from build123d import *

# Parameters (mm, degrees)
SKETCH002_W  = 4
SKETCH002_H  = 3
PAD002_DEPTH = 4
SKETCH_W     = 2
SKETCH_H     = 4
PAD_DEPTH    = 6


with BuildPart() as part:
    # Sketch002 → Pad002 (new body)
    with BuildSketch(Plane.XZ.offset(-2)):
        Polygon((3.75, 0), (3.75, 22), (3.75, 22), (2.25, 22), (-3.75, 22), (-3.75, 0), (-3.75, -3.5), (6.25, -3.5), (6.25, -1.5), (-1.75, -1.5), (-1.75, 0), align=None)
        with Locations((0.25, 16.5)):
            Rectangle(SKETCH002_W, SKETCH002_H, mode=Mode.SUBTRACT)
    extrude(amount=PAD002_DEPTH)

    # Sketch (on Pad) → Pad (join)
    with BuildSketch(Plane.XZ.offset(-2)):
        with Locations((-2.75, 13)):
            Rectangle(SKETCH_W, SKETCH_H)
    pad = extrude(amount=PAD_DEPTH)

    # Mirrored: Pad across XZ
    add(pad.mirror(Plane.XZ))


solid = part.part
The model under review builds one solid part; all positions refer to its coordinate system, in mm. A direction names the side the tool comes from. Round coordinates to 2 decimals unless told otherwise and drop trailing zeros. Loops run counter-clockwise (first coordinate to the right, second up) from the corner with the lowest first, then second, coordinate; pieces in that order, holes last. Notation, with made-up numbers: M 54.5,-7 L 108.5,-7 A30 ccw 108.5,19 Z; hole C -2,-15 d2. An arc over 180 degrees is marked long. Answer as a JSON object with one key per item and string values.
Item 1: For line 1 along X through (y, z) = (1.5, 17.25); line 2 along Z through (x, y) = (0.75, 0); line 3 along X through (y, z) = (0.5, 19.25), list the stretches that pass through material, from the lowest coordinate up.
Check sheet entries:
{"line 1": "-3.75 to -1.75, 2.25 to 3.75", "line 2": "-3.5 to -1.5, 0 to 15, 18 to 22", "line 3": "-3.75 to 3.75"}
Item 2: We need section A-A, the plane x = -1. State the section outline as (y, z) points, and give its area (3 significant figures).
Check sheet entries:
{"outline": "M -2,-3.5 L 2,-3.5 L 2,-1.5 L -2,-1.5 Z; M -2,0 L 2,0 L 2,15 L -2,15 Z; M -2,18 L 2,18 L 2,22 L -2,22 Z", "area": "84.0 mm2"}
Item 3: We need section B-B, the plane y = -0.75. State the section outline as (x, z) points, and give its area (3 significant figures).
Check sheet entries:
{"outline": "M -3.75,-3.5 L 6.25,-3.5 L 6.25,-1.5 L -1.75,-1.5 L -1.75,0 L 3.75,0 L 3.75,22 L -3.75,22 Z; hole M -1.75,15 L 2.25,15 L 2.25,18 L -1.75,18 Z", "area": "176 mm2"}
Item 4: Clearance check with flat-ended pins moving along their axes: P1, Ø0.8, axis at y = -0.5, z = -1, coming from the +X side; P2, Ø3, axis at x = -2, z = -1, coming from the +Y side; P3, Ø3, axis at x = 1, z = 6, coming from the -Y side. State where each tip first meets the part, or that it passes through.
Check sheet entries:
{"P1": "x = -1.75", "P2": "y = 2", "P3": "y = -2"}
Item 5: We need section D-D, the plane z = 14.25. State the section outline as (x, y) points, and give its area (3 significant figures).
Check sheet entries:
{"outline": "M -3.75,-4 L -1.75,-4 L -1.75,-2 L 3.75,-2 L 3.75,2 L -1.75,2 L -1.75,4 L -3.75,4 Z", "area": "38.0 mm2"}
Item 6: The part is to be moulded in two halves that separate along Z. For faces 6 (the face through (-3, 3, 11)), 7 (the face through (-3, 4, 13)), 8 (the face through (0, 0, 15)), 9 (the face through (0, 0, 22)), say which applies: +Z half, -Z half, draft (parallel to the pull), parting line (faces both ways), or undercut.
Check sheet entries:
{"face 6": "-Z half", "face 7": "draft", "face 8": "undercut", "face 9": "+Z half"}
Item 7: We need section C-C, the plane x = -2. State the section outline as (y, z) points.
Check sheet entries:
{"outline": "M -4,11 L -2,11 L -2,-3.5 L 2,-3.5 L 2,11 L 4,11 L 4,15 L 2,15 L 2,22 L -2,22 L -2,15 L -4,15 Z"}
Item 8: Tool access review of faces 1 (the face through (-1.75, -3, 13)), 2 (the face through (2, 0, -1.5)), 3 (the face through (3.75, 0, 11)), 4 (the face through (-1.75, 3, 13)), 5 (the face through (2.25, 0, 16)): name each direction out of +Z, -Z, +X, -X, +Y, -Y from which nothing blocks a thin tool from reaching the whole face with its end or side.
Check sheet entries:
{"face 1": "+Z, -Z, +X, -Y", "face 2": "+X, +Y, -Y", "face 3": "+Z, +X, +Y, -Y", "face 4": "+Z, -Z, +X, +Y", "face 5": "+Y, -Y"}
